```python
from build123d import *

# Parameters (mm, degrees)
SKETCH1_W           = 91
SKETCH1_H           = 70
BOSS_EXTRUDE1_DEPTH = 12
SKETCH2_R           = 2
CUT_EXTRUDE1_DEPTH  = 59.645119149
SKETCH4_W           = 6.2
SKETCH4_H           = 6.2
CUT_EXTRUDE2_DEPTH  = 15
SKETCH5_W           = 70
SKETCH5_H           = 42
CUT_EXTRUDE3_DEPTH  = 6.2
SKETCH6_W           = 109.081458423
SKETCH6_H           = 97.427456455
SKETCH6_W_2         = 85
SKETCH6_H_2         = 75.166710869
CUT_EXTRUDE4_DEPTH  = 28
SKETCH7_W           = 85
SKETCH7_H           = 3.5
CUT_EXTRUDE5_DEPTH  = 82.081748871
FILLET3_R           = 10
SKETCH8_W           = 85
SKETCH8_H           = 10
CUT_EXTRUDE7_DEPTH  = 17


with BuildPart() as part:
    # Sketch1 → Boss-Extrude1 (new body)
    with BuildSketch(Plane(origin=(0, 0, 0), x_dir=(1, 0, 0), z_dir=(0, 1, 0))):
        Rectangle(SKETCH1_W, SKETCH1_H)
    extrude(amount=BOSS_EXTRUDE1_DEPTH)

    # Sketch2 → Cut-Extrude1 (cut, through all)
    with BuildSketch(Plane(origin=(0, 12, 0), x_dir=(1, 0, 0), z_dir=(0, 1, 0))):
        with Locations(Location((-20.5, -4, 0), (0, 0, 270))):
            Circle(SKETCH2_R)
        with Locations(Location((20.5, -4, 0), (0, 0, 270))):
            Circle(SKETCH2_R)
    extrude(amount=-CUT_EXTRUDE1_DEPTH, mode=Mode.SUBTRACT)

    # Sketch4 → Cut-Extrude2 (cut)
    with BuildSketch(Plane(origin=(0, 0, -35), x_dir=(-1, 0, 0), z_dir=(0, 0, -1))):
        with Locations((-12.4, 8.9)):
            Rectangle(SKETCH4_W, SKETCH4_H)
        with Locations((12.4, 8.9)):
            Rectangle(SKETCH4_W, SKETCH4_H)
    extrude(amount=-CUT_EXTRUDE2_DEPTH, mode=Mode.SUBTRACT)

    # Sketch5 → Cut-Extrude3 (cut)
    with BuildSketch(Plane(origin=(0, 12, 0), x_dir=(1, 0, 0), z_dir=(0, 1, 0))):
        with Locations((0, 4)):
            Rectangle(SKETCH5_W, SKETCH5_H)
    extrude(amount=-CUT_EXTRUDE3_DEPTH, mode=Mode.SUBTRACT)

    # Sketch6 → Cut-Extrude4 (cut)
    with BuildSketch(Plane(origin=(0, 12, 0), x_dir=(1, 0, 0), z_dir=(0, 1, 0))):
        with Locations((-1.57183243, 4.07575105)):
            Rectangle(SKETCH6_W, SKETCH6_H)
        with Locations((0, 4.583355434)):
            Rectangle(SKETCH6_W_2, SKETCH6_H_2, mode=Mode.SUBTRACT)
    extrude(amount=-CUT_EXTRUDE4_DEPTH, mode=Mode.SUBTRACT)

    # Sketch7 → Cut-Extrude5 (cut, through all)
    with BuildSketch(Plane(origin=(0, 0, -35), x_dir=(-1, 0, 0), z_dir=(0, 0, -1))):
        with Locations((0, 1.75)):
            Rectangle(SKETCH7_W, SKETCH7_H)
    extrude(amount=-CUT_EXTRUDE5_DEPTH, mode=Mode.SUBTRACT)

    # Fillet3
    # the kernel refuses this fillet: 10 mm, written as the material it takes off along each edge
    with BuildSketch(Plane(origin=(-67.217149917, 3.5, 33), x_dir=(0, 0, -1), z_dir=(1, 0, 0))) as fillet3_piece_1:
        with BuildLine():
            CenterArc((9.886859967, 10), FILLET3_R, 188.626926559, 81.373073441)
            Line((0, 8.5), (-0.197737199, 8.47))
            ThreePointArc((-0.197737199, 8.47), (-0.2, 4.25), (-0.2, 0))
            Line((-0.2, 0), (0, -0.2))
            Line((0, -0.2), (9.886859967, -0.2))
            Line((9.886859967, -0.2), (9.886859967, 0))
        make_face()
    extrude(amount=134.434299833, mode=Mode.SUBTRACT)

    # Sketch8 → Cut-Extrude7 (cut)
    with BuildSketch(Plane(origin=(0, 12, 0), x_dir=(1, 0, 0), z_dir=(0, 1, 0))):
        with Locations((0, -28)):
            Rectangle(SKETCH8_W, SKETCH8_H)
    extrude(amount=-CUT_EXTRUDE7_DEPTH, mode=Mode.SUBTRACT)


solid = part.part
```
Verification items for the finished model (mm, model axes). A direction names the side the tool comes from. Coordinates: 2 decimals unless noted, no trailing zeros. Write each loop counter-clockwise with the first axis right and the second up, starting at its lowest first coordinate (ties: lowest second). Pieces come first, ordered by that corner, then holes. Notation, with made-up numbers: M -3,-35.5 L 20,-35.5 A28 cw 20,-0.5 Z; hole C 30,88 d1. An arc over 180 degrees is marked long. Answer as a JSON object with one key per item and string values. Group by question number.
(1) Release check for a two-part mould opening along X. For faces 1 (the face through (-1, 8, -35)), 2 (the face through (-9.3, 9, -30)), 3 (the face through (-42.5, 8, -6)) record: +X half, -X half, draft (parallel to the pull), parting line (faces both ways), or undercut.
(2) Cross-section at B-B, the plane z = 4. Record the cut outline in (x, y).
(3) Tool access check on faces 4 (the face through (-18.517, 4.666, 3.74)), 5 (the face through (15.5, 9, -30)), 6 (the face through (0, 9, -25)). Record the directions out of +Z, -Z, +X, -X, +Y, -Y that give a thin tool (end or side, any length) a straight path to the whole face; none if there is none.
(4) Cross-section at C-C, the plane y = 9.25. Record the cut outline in (x, z).
(5) Cross-section at A-A, the plane x = -20.5. Record the cut outline in (y, z), and give its area (3 significant figures).
(6) Material ranges on line 1 (X direction, y = 10.5, z = -29); line 2 (X direction, y = 4.95, z = 4); line 3 (Z direction, x = 29, y = 10), recorded low to high.
(7) Cross-section at D-D, the plane x = 3. Record the cut outline in (y, z).
(8) Gauge pin test, flat ends, axial feed: pin 1 (3 mm diameter, centred on x = -25.5, z = -14, fed in from +Y); pin 2 (3 mm diameter, centred on x = -20.5, z = 4, fed in from -Y). Record the tip position at first contact, or that the pin passes through.
Reply:
{
 "1": {"face 1": "draft", "face 2": "undercut", "face 3": "-X half"},
 "2": {"outline": "M -42.5,3.5 L -22.5,3.5 L -22.5,5.8 L -35,5.8 L -35,12 L -42.5,12 Z; M -18.5,3.5 L 18.5,3.5 L 18.5,5.8 L -18.5,5.8 Z; M 22.5,3.5 L 42.5,3.5 L 42.5,12 L 35,12 L 35,5.8 L 22.5,5.8 Z"},
 "3": {"face 4": "+Y, -Y", "face 5": "-Z, +Y", "face 6": "+Y"},
 "4": {"outline": "M -42.5,-35 L -15.5,-35 L -15.5,-25 L -35,-25 L -35,17 L 35,17 L 35,-25 L 15.5,-25 L 15.5,-35 L 42.5,-35 L 42.5,23 L -42.5,23 Z; M -9.3,-35 L 9.3,-35 L 9.3,-25 L -9.3,-25 Z"},
 "5": {"outline": "M 3.5,-35 L 12,-35 L 12,-25 L 5.8,-25 L 5.8,2 L 3.5,2 Z; M 3.5,6 L 5.8,6 L 5.8,17 L 12,17 L 12,23 L 3.5,23 Z", "area": "223 mm²"},
 "6": {"line 1": "-42.5 to -15.5, -9.3 to 9.3, 15.5 to 42.5", "line 2": "-42.5 to -22.5, -18.5 to 18.5, 22.5 to 42.5", "line 3": "-35 to -25, 17 to 23"},
 "7": {"outline": "M 3.5,-35 L 12,-35 L 12,-25 L 5.8,-25 L 5.8,17 L 12,17 L 12,23 L 3.5,23 Z"},
 "8": {"pin 1": "y = 5.8", "pin 2": "through"}
}
